Read the model definition and answer for the solid it produces. Units are mm, in the model's axes. A direction names the side the tool comes from. Give positions to 0.01 mm unless a question says otherwise; leave off trailing zeros. Write each loop counter-clockwise with the first axis right and the second up, starting at its lowest first coordinate (ties: lowest second). Pieces come first, ordered by that corner, then holes. Notation, with made-up numbers: M 88.25,53 L 96.25,53 A11 cw 96.25,62 Z; hole C 69,-33 d1. An arc over 180 degrees is marked long. Use a Markdown table: item, result. Add a question column.
Item 1: A cutting plane is placed at D-D on y = 75.65. Determine the outline of the cut face in (x, z), then the cut area to 3 significant figures.
Item 2: The mould has two halves that part along Y. Classify faces 4 (the cylindrical face through (27.045, 1.795, -5.562)), 5 (the cylindrical face through (19.47, 81.5, 5.08)), 6 (the flat face through (-5, 60, 2)): pulls with the +Y half, pulls with the -Y half, needs draft (parallel to the pull), parting line crosses it, or undercut.
Item 3: Given P1, Ø1.5, axis at x = -7.5, y = 61, coming from the -Z side; P2, Ø7.5, axis at x = -25, z = 2, coming from the +Y side; P3, Ø6, axis at y = 42.5, z = 3.5, coming from the -X side; P4, Ø2.5, axis at x = -15.55, y = 44.54, coming from the +Z side, each flat-ended and moving along its own axis, determine where each tip first touches the part or whether it passes through.
Item 4: A cutting plane is placed at A-A on x = 28.9. Determine the outline of the cut face in (y, z), then the cut area to 3 significant figures.
Item 5: A cutting plane is placed at C-C on z = -5.15. Determine the outline of the cut face in (x, y).
Item 6: For faces 1 (the flat face through (20.9, 33, 2)), 2 (the flat face through (-20.9, 34, 2)), 3 (the flat face through (0, 37.1, -5)), determine the directions among +Z, -Z, +X, -X, +Y, -Y from which every point of the face is accessible in a straight line to the end or side of a thin tool.
Item 7: A cutting plane is placed at B-B on y = 60.1. Determine the outline of the cut face in (x, z).
Item 8: Consider probe 1 along X at (y, z) = (1.6, 5.15); probe 2 along X at (y, z) = (75.5, 9); probe 3 along Z at (x, y) = (28.9, 1.1). Determine where each line is inside the solid, lowest interval first. Write a range as [from, to].
from build123d import *

# Parameters (mm, degrees)
IZIM1_R                                            = 4
IZIM1_R_2                                          = 1.45
Y_KSEKLIK_EKSTR_ZYON1_DEPTH                        = 10.3
IZIM2_R                                            = 1.9
KES_EKSTR_ZYON1_DEPTH                              = 10.3
M3_ALT_GEN_ALYAN_HAV_A_BA_L_K_R_VIDA_I_D           = 3.6
M3_ALT_GEN_ALYAN_HAV_A_BA_L_K_R_VIDA_I_CSINK_D     = 6.72
M3_ALT_GEN_ALYAN_HAV_A_BA_L_K_R_VIDA_I_CSINK_ANGLE = 90
IZIM4_R                                            = 11
KES_EKSTR_ZYON2_DEPTH                              = 2
Y_KSEKLIK_EKSTR_ZYON2_DEPTH                        = 10.3
IZIM6_R                                            = 1.9
KES_EKSTR_ZYON3_DEPTH                              = 10.3
M3_ALT_GEN_ALYAN_HAV_A_BA_L_K_R_VID_2_D            = 3.6
M3_ALT_GEN_ALYAN_HAV_A_BA_L_K_R_VID_2_CSINK_D      = 6.72
M3_ALT_GEN_ALYAN_HAV_A_BA_L_K_R_VID_2_CSINK_ANGLE  = 90


with BuildPart() as part:
    # Çizim1 → Yükseklik-Ekstrüzyon1 (new body)
    with BuildSketch(Plane.XY):
        with BuildLine():
            Line((-35.9, 0), (35.9, 0))
            Line((35.9, 0), (35.9, 5))
            Line((35.9, 5), (20.9, 5))
            Line((20.9, 5), (20.9, 78))
            ThreePointArc((20.9, 78), (19.435533906, 81.535533906), (15.9, 83))
            Line((15.9, 83), (-15.9, 83))
            ThreePointArc((-15.9, 83), (-19.435533906, 81.535533906), (-20.9, 78))
            Line((-20.9, 78), (-20.9, 5))
            Line((-20.9, 5), (-35.9, 5))
            Line((-35.9, 5), (-35.9, 0))
        make_face()
        with Locations(Location((0, 60.1, 0), (0, 0, 180))):
            Circle(IZIM1_R, mode=Mode.SUBTRACT)
        with Locations(Location((-15.55, 75.65, 0), (0, 0, 180))):
            Circle(IZIM1_R_2, mode=Mode.SUBTRACT)
        with Locations(Location((15.56, 75.65, 0), (0, 0, 180))):
            Circle(IZIM1_R_2, mode=Mode.SUBTRACT)
        with Locations(Location((15.56, 44.54, 0), (0, 0, 180))):
            Circle(IZIM1_R_2, mode=Mode.SUBTRACT)
        with Locations(Location((-15.55, 44.54, 0), (0, 0, 180))):
            Circle(IZIM1_R_2, mode=Mode.SUBTRACT)
    extrude(amount=Y_KSEKLIK_EKSTR_ZYON1_DEPTH)

    # Çizim2 → Kes-Ekstrüzyon1 (cut)
    with BuildSketch(Plane(origin=(0, 5, 0), x_dir=(1, 0, 0), z_dir=(0, 1, 0))):
        with Locations(Location((28.9, -5.15, 0), (0, 0, 270))):
            Circle(IZIM2_R)
        with Locations(Location((-28.9, -5.15, 0), (0, 0, 270))):
            Circle(IZIM2_R)
    extrude(amount=-KES_EKSTR_ZYON1_DEPTH, mode=Mode.SUBTRACT)

    # M3 Alt_gen Alyan Hav_a Ba_l_ K_r Vida _i (through all)
    with Locations(Plane(origin=(-28.9, 5, 5.15), x_dir=(0, 0, 1), z_dir=(0, 1, 0))):
        with Locations((0, 0), (0, 57.8)):
            CounterSinkHole(M3_ALT_GEN_ALYAN_HAV_A_BA_L_K_R_VIDA_I_D / 2, M3_ALT_GEN_ALYAN_HAV_A_BA_L_K_R_VIDA_I_CSINK_D / 2, counter_sink_angle=M3_ALT_GEN_ALYAN_HAV_A_BA_L_K_R_VIDA_I_CSINK_ANGLE)

    # Çizim4 → Kes-Ekstrüzyon2 (cut)
    with BuildSketch(Plane(origin=(0, 0, 0), x_dir=(-1, 0, 0), z_dir=(0, 0, -1))):
        with Locations((0, 60.1)):
            Circle(IZIM4_R)
    extrude(amount=-KES_EKSTR_ZYON2_DEPTH, mode=Mode.SUBTRACT)

    # Çizim5 → Yükseklik-Ekstrüzyon2 (add)
    with BuildSketch(Plane(origin=(0, 0, 0), x_dir=(-1, 0, 0), z_dir=(0, 0, -1))):
        Polygon((-20.9, 37.1), (20.9, 37.1), (20.9, 5), (35.9, 5), (35.9, 0), (-35.9, 0), (-35.9, 5), (-20.9, 5), align=None)
    extrude(amount=Y_KSEKLIK_EKSTR_ZYON2_DEPTH)

    # Çizim6 → Kes-Ekstrüzyon3 (cut)
    with BuildSketch(Plane(origin=(0, 5, 0), x_dir=(1, 0, 0), z_dir=(0, 1, 0))):
        with Locations(Location((28.9, 5.15, 0), (0, 0, 270))):
            Circle(IZIM6_R)
        with Locations(Location((-28.9, 5.15, 0), (0, 0, 270))):
            Circle(IZIM6_R)
    extrude(amount=-KES_EKSTR_ZYON3_DEPTH, mode=Mode.SUBTRACT)

    # M3 Alt_gen Alyan Hav_a Ba_l_ K_r Vid 2 (through all)
    with Locations(Plane(origin=(-28.9, 5, -5.15), x_dir=(0, 0, 1), z_dir=(0, 1, 0))):
        with Locations((0, 0), (0, 57.8)):
            CounterSinkHole(M3_ALT_GEN_ALYAN_HAV_A_BA_L_K_R_VID_2_D / 2, M3_ALT_GEN_ALYAN_HAV_A_BA_L_K_R_VID_2_CSINK_D / 2, counter_sink_angle=M3_ALT_GEN_ALYAN_HAV_A_BA_L_K_R_VID_2_CSINK_ANGLE)


solid = part.part
Filled in:
| question | item | result |
|---|---|---|
| 1 | outline | M -20.9,0 L -17,0 L -17,10.3 L -20.9,10.3 Z; M -14.1,0 L 14.11,0 L 14.11,10.3 L -14.1,10.3 Z; M 17.01,0 L 20.9,0 L 20.9,10.3 L 17.01,10.3 Z |
| 1 | area | 371 mm² |
| 2 | face 4 | needs draft |
| 2 | face 5 | pulls with the +Y half |
| 2 | face 6 | undercut |
| 3 | P1 | z = 2 |
| 3 | P2 | y = 5 |
| 3 | P3 | x = -20.9 |
| 3 | P4 | through |
| 4 | outline | M 0,-10.3 L 5,-10.3 L 5,-8.51 L 3.54,-7.05 L 0,-7.05 Z; M 0,-3.25 L 3.54,-3.25 L 5,-1.79 L 5,1.79 L 3.54,3.25 L 0,3.25 Z; M 0,7.05 L 3.54,7.05 L 5,8.51 L 5,10.3 L 0,10.3 Z |
| 4 | area | 60.7 mm² |
| 5 | outline | M -35.9,0 L -30.8,0 L -30.8,3.54 L -32.26,5 L -35.9,5 Z; M -27,0 L 27,0 L 27,3.54 L 25.54,5 L 20.9,5 L 20.9,37.1 L -20.9,37.1 L -20.9,5 L -25.54,5 L -27,3.54 Z; M 30.8,0 L 35.9,0 L 35.9,5 L 32.26,5 L 30.8,3.54 Z |
| 6 | face 1 | +Z, -Z, +X, +Y |
| 6 | face 2 | +Z, -Z, -X, +Y |
| 6 | face 3 | -Z, +X, -X, +Y |
| 7 | outline | M -20.9,0 L -11,0 L -11,2 L -4,2 L -4,10.3 L -20.9,10.3 Z; M 4,2 L 11,2 L 11,0 L 20.9,0 L 20.9,10.3 L 4,10.3 Z |
| 8 | probe 1 | [-35.9, -30.8], [-27, 27], [30.8, 35.9] |
| 8 | probe 2 | [-20.9, -16.99], [-14.11, 14.12], [17, 20.9] |
| 8 | probe 3 | [-10.3, -7.05], [-3.25, 3.25], [7.05, 10.3] |
